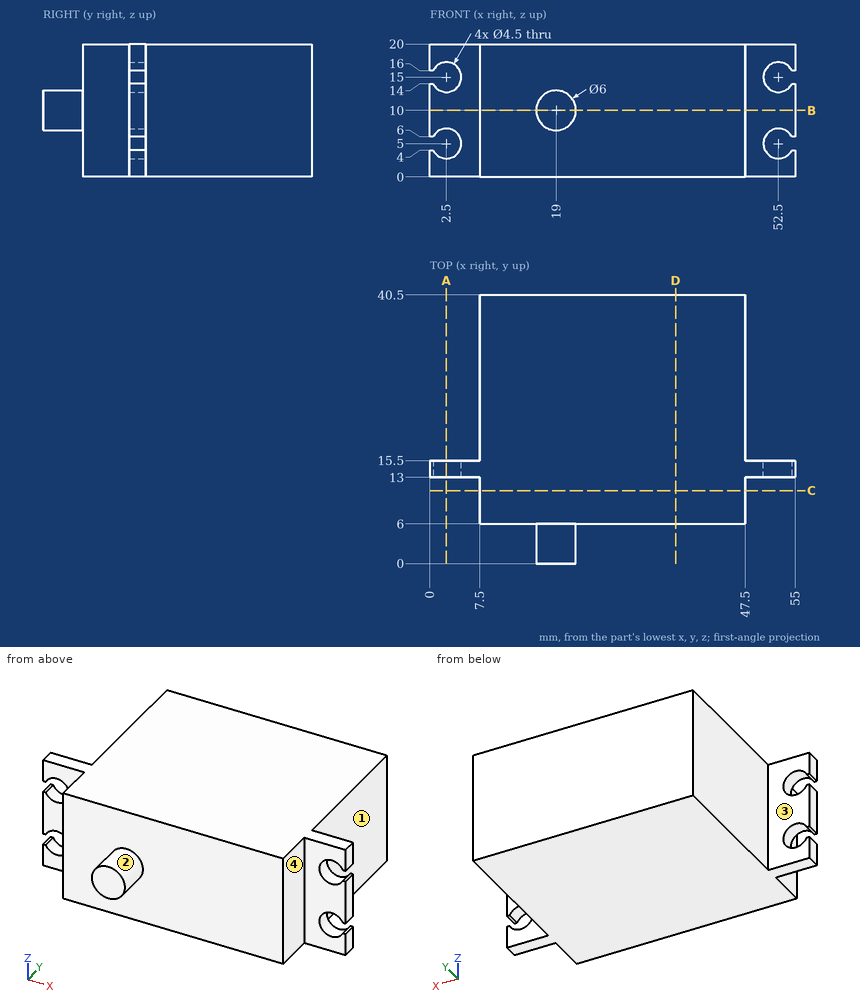
Input: dimensioned drawing with shaded views. Units: mm. Origin: part minimum x, y, z. A direction names the side the tool comes from. Coordinates: 2 decimals unless noted, no trailing zeros. Loops run counter-clockwise (first coordinate to the right, second up) from the corner with the lowest first, then second, coordinate; pieces in that order, holes last. Notation, with made-up numbers: M 42,66 L 82,66 A16 ccw 82,87 Z; hole C -9,57.5 d1. An arc over 180 degrees is marked long. Use a Markdown table: item, result. Add a question column.
Q1. First-contact query: pin 1 (4 mm diameter, centred on x = 5, z = 10.5, fed in from +Y); pin 2 (8 mm diameter, centred on x = 51, z = 10.5, fed in from -Y); pin 3 (10 mm diameter, centred on x = 49, z = 18, fed in from +Y); pin 4 (4 mm diameter, centred on y = 7.5, z = 7.5, fed in from +X). Flat tips, straight axial feed; report the tip coordinate or a pass-through.
Q2. Material intervals for L1, parallel to Z at x = 2.5, y = 13.85; L2, parallel to X at y = 20, z = 10.25; L3, parallel to Y at x = 44, z = 11.25, sorted ascending.
Q3. Section query D-D, the plane x = 37. Return loops of the section in (y, z).
Q4. Section query A-A, the plane x = 2.5. Return loops of the section in (y, z), and give its area (3 significant figures).
Q5. Section query C-C, the plane y = 11. Return loops of the section in (x, z).
Q6. Section query B-B, the plane z = 10. Return loops of the section in (x, y), and give its area (3 significant figures).
Q7. Access query for the marked faces 1, 2, 3 and 4. Directions: +Z, -Z, +X, -X, +Y, -Y. A direction counts if a zero-diameter tool reaches every point of the face in a straight line with its end or side. Return the directions, or none.
Result:
| question | item | result |
|---|---|---|
| 1 | pin 1 | stops at y = 15.5 |
| 1 | pin 2 | stops at y = 6 |
| 1 | pin 3 | stops at y = 40.5 |
| 1 | pin 4 | stops at x = 47.5 |
| 2 | L1 | z = 0 to 2.75, 7.25 to 12.75, 17.25 to 20 |
| 2 | L2 | x = 7.5 to 47.5 |
| 2 | L3 | y = 6 to 40.5 |
| 3 | outline | M 6,0 L 40.5,0 L 40.5,20 L 6,20 Z |
| 4 | outline | M 13,0 L 15.5,0 L 15.5,2.75 L 13,2.75 Z; M 13,7.25 L 15.5,7.25 L 15.5,12.75 L 13,12.75 Z; M 13,17.25 L 15.5,17.25 L 15.5,20 L 13,20 Z |
| 4 | area | 27.5 mm2 |
| 5 | outline | M 7.5,0 L 47.5,0 L 47.5,20 L 7.5,20 Z |
| 6 | outline | M 0,13 L 7.5,13 L 7.5,6 L 16,6 L 16,0 L 22,0 L 22,6 L 47.5,6 L 47.5,13 L 55,13 L 55,15.5 L 47.5,15.5 L 47.5,40.5 L 7.5,40.5 L 7.5,15.5 L 0,15.5 Z |
| 6 | area | 1,450 mm2 |
| 7 | face 1 | +Z, -Z, +X, +Y |
| 7 | face 2 | -Y |
| 7 | face 3 | +Z, -Z, -X, +Y |
| 7 | face 4 | +Z, -Z, +X, -Y |
